Source: CAD feature listing. Evaluate the final solid. Frame: model axes, mm. A direction names the side the tool comes from. Give positions to 0.01 mm unless a question says otherwise; leave off trailing zeros. Loops run counter-clockwise (first coordinate to the right, second up) from the corner with the lowest first, then second, coordinate; pieces in that order, holes last. Notation, with made-up numbers: M 11,11 L 44,11 A11 cw 44,19 Z; hole C 7,42 d2. An arc over 180 degrees is marked long. Answer in a Markdown table with one row per item.
```python
from build123d import *


with BuildPart() as part:
    # Sketch5 → Revolve1 (revolve)
    with BuildSketch(Plane(origin=(0, 0, 0), x_dir=(0, 0, -1), z_dir=(1, 0, 0))):
        with BuildLine():
            Line((0, 0), (0, 3))
            ThreePointArc((0, 3), (0.292893219, 3.707106781), (1, 4))
            Line((1, 4), (15, 4))
            Line((15, 4), (15, 5.5))
            Line((15, 5.5), (16, 5.5))
            Line((16, 5.5), (16, 2))
            Line((16, 2), (21.5, 2))
            Line((21.5, 2), (24.738971507, 0.426455304))
            ThreePointArc((24.738971507, 0.426455304), (25.24442356, 0.436184735), (25.5, 0))
            Line((25.5, 0), (0, 0))
        make_face()
    revolve(axis=Axis((0, 0, 0), (0, 0, -1)))


solid = part.part
```
Q1. Ray query, probe 1 along Z at (x, y) = (2.5, -4); probe 2 along Z at (x, y) = (-1.75, 2.25); probe 3 along Y at (x, z) = (2.5, -11.25). Return the intervals inside material, ascending. Write a range as from..to.
Values follow:
| item | result |
|---|---|
| probe 1 | -16..-15 |
| probe 2 | -16..0 |
| probe 3 | -3.12..3.12 |
Q2. Reachability of faces 1 (the flat face through (-2, 4, -15)), 2 (the cylindrical face through (-2, 0, -19)), 3 (the cylindrical face through (-5.37, -1.19, -15.51)) from +Z, -Z, +X, -X, +Y, -Y: full face, straight path, thin tool, end or side. Return the list, or none.
Values follow:
| item | result |
|---|---|
| face 1 | +Z |
| face 2 | -Z |
| face 3 | +Z, -Z |
Q3. Section query B-B (z = -18.5). Output: boundary loops of the cut face in (x, y).
Values follow:
| item | result |
|---|---|
| outline | C 0,0 d4 |
Q4. Contact query for flat-ended pins moving along their axis: pin 1 Ø4 at (x, y) = (-2.5, -4) entering from -Z; pin 2 Ø1 at (y, z) = (1.5, -12.5) entering from -X; pin 3 Ø3 at (y, z) = (0.5, -4) entering from -X. Output: stop coordinate, or through.
Values follow:
| item | result |
|---|---|
| pin 1 | z = -16 |
| pin 2 | x = -3.87 |
| pin 3 | x = -4 |
Q5. Section query D-D (z = -13). Output: boundary loops of the cut face in (x, y).
Values follow:
| item | result |
|---|---|
| outline | C 0,0 d8 |
Q6. Section query A-A (y = 0). Output: boundary loops of the cut face in (x, z).
Values follow:
| item | result |
|---|---|
| outline | M -5.5,-16 L -2,-16 L -2,-21.5 L -0.43,-24.74 A0.5 ccw long 0.43,-24.74 L 2,-21.5 L 2,-16 L 5.5,-16 L 5.5,-15 L 4,-15 L 4,-1 A1 ccw 3,0 L -3,0 A1 ccw -4,-1 L -4,-15 L -5.5,-15 Z |
